Autodesk Fusion 360 part; units mm, degrees
sketch "Sketch1" plane through (0, 0, 0) normal (0, 1, 0) x (1, 0, 0)
  circle A0 centre (0, 0) radius 4
  dimension "d1" = 8
extrude "Extrude1" add sketch "Sketch1" along normal blind 200
sketch "Sketch2" plane through (0, 0, 0) normal (1, 0, 0) x (0, 0, -1)
  circle A0 centre (0, 4.5) radius 1.245
  circle A1 centre (0, 9.5) radius 1.245
  line L0 (4, 0) -> (-4, 0)
  line L1 (0, 0) -> (0, 13) construction
  dimension "d4" = 2.49
  dimension "d5" = 5
  dimension "d6" = 4.5
extrude "Extrude2" cut sketch "Sketch2" along normal through all and the other way through all
Model file for the job. Use its own axes, mm. Coordinates: 2 decimals unless noted, no trailing zeros. Loops run counter-clockwise (first coordinate to the right, second up) from the corner with the lowest first, then second, coordinate; pieces in that order, holes last. Notation, with made-up numbers: (54.25, 26) -> (113.25, 26) arc R16 cw to (113.25, 39) -> close; hole circle Ø3 at (9.5, -18). An arc over 180 degrees is marked (long way). Use one line per item in the form item = value. Start each with the question number.
(1) Cut at B-B on x = -2.5. Give the cut face in (y, z) (1 decimal).
(2) Cut at A-A on z = 0. Give the cut face in (x, y) (3 decimals).
(3) Cut at C-C on y = 101. Give the cut face in (x, z), and give its area (3 significant figures).
(4) Probe probe 1 along Y at (x, z) = (1.75, 0) (3 decimals); probe 2 along Y at (x, z) = (-3, -0.75); probe 3 along Z at (x, y) = (-2, 9.5) (3 decimals). List the from-to ranges inside material, lowest first. Write a range as from..to.
(5) Flat gauge pins, fed straight in: pin 1 (2 mm diameter, centred on x = 1.5, y = 51.5, fed in from +Z); pin 2 (2 mm diameter, centred on x = -2, y = 87, fed in from -Z). Where does each tip first touch, or does it go through?
Values:
q1.outline = (0, -3.1) -> (200, -3.1) -> (200, 3.1) -> (0, 3.1) -> close; hole circle Ø2.5 at (4.5, 0); hole circle Ø2.5 at (9.5, 0)
q2.outline = (-4, 0) -> (4, 0) -> (4, 3.255) -> (-4, 3.255) -> close; (-4, 5.745) -> (4, 5.745) -> (4, 8.255) -> (-4, 8.255) -> close; (-4, 10.745) -> (4, 10.745) -> (4, 200) -> (-4, 200) -> close
q3.outline = circle Ø8 at (0, 0)
q3.area = 50.3 mm2
q4.probe_1 = 0..3.255, 5.745..8.255, 10.745..200
q4.probe_2 = 0..3.51, 5.49..8.51, 10.49..200
q4.probe_3 = -3.464..-1.245, 1.245..3.464
q5.pin_1 = 3.97
q5.pin_2 = -3.87
